Autodesk Inventor part; units mm, degrees
ref_plane "YZ Plane" through (0, 0, 0) normal (1, 0, 0) x (0, 1, 0)
ref_plane "XZ Plane" through (0, 0, 0) normal (0, 1, 0) x (-1, 0, 0)
ref_plane "XY Plane" through (0, 0, 0) normal (0, 0, 1) x (1, 0, 0)
sketch "Sketch1" plane through (0, 0, 0) normal (0, 0, 1) x (1, 0, 0)
  line L0 (0, 0) -> (-1016, 0)
  line L1 (-1016, 0) -> (-1016, 1016)
  line L2 (-1016, 1016) -> (0, 1016)
  line L3 (0, 1016) -> (0, 0)
  line L4 (19.05, 1035.05) -> (-1035.05, 1035.05)
  line L5 (-1035.05, 1035.05) -> (-1035.05, -19.05)
  line L6 (-1035.05, -19.05) -> (19.05, -19.05)
  line L7 (19.05, -19.05) -> (19.05, 1035.05)
  line L8 (-685.8, 1016) -> (-685.8, 1035.05)
  line L9 (-330.2, 1016) -> (-330.2, 1035.05)
  line L10 (-685.8, -19.05) -> (-685.8, 0)
  line L11 (-330.2, -19.05) -> (-330.2, 0)
  line L12 (0, 330.2) -> (19.05, 330.2)
  line L13 (0, 685.8) -> (19.05, 685.8)
  line L14 (-1016, 685.8) -> (-1035.05, 685.8)
  line L15 (-1016, 330.2) -> (-1035.05, 330.2)
  point P0 (-1644.65, 1016)
  point P1 (-1644.65, 1035.05)
  point P2 (-387.35, 1016)
  point P3 (-387.35, 1035.05)
  point P4 (-685.8, -19.05)
  point P5 (-685.8, 0)
  point P6 (-330.2, 0)
  point P7 (-330.2, -19.05)
  dimension "d0" = 1016
  dimension "d1" = 1016
  dimension "d2" = 19.05
  dimension "d5" = 355.6
  dimension "d7" = 355.6
  dimension "d10" = 349.25
  dimension "d11" = 349.25
  dimension "d12" = 355.6
  dimension "d13" = 349.25
  dimension "d14" = 349.25
  dimension "d15" = 349.25
  dimension "d18" = 349.25
extrude "Extrusion1" add sketch "Sketch1" along normal blind 19.05 contours L0 L1 L2 L3 | L11 L6 L10 L0 | L3 L13 L7 L12 | L15 L5 L14 L1 | L2 L8 L4 L9
properties part number "Final Product backplate"
Read the model definition and answer for the solid it produces. Units are mm, in the model's axes. Coordinates: 2 decimals unless noted, no trailing zeros. Loops run counter-clockwise (first coordinate to the right, second up) from the corner with the lowest first, then second, coordinate; pieces in that order, holes last.
Q1. Consider probe 1 along Y at (x, z) = (-134.5, 5.5); probe 2 along X at (y, z) = (924.5, 6.5). Determine where each line is inside the solid, lowest interval first.
Q2. The part is cut by section B-B on x = -757.5. Write down the section's boundary in (y, z).
Q3. The part is cut by section A-A on z = 12. Write down the section's boundary in (x, y).
Q4. Each of these flat-tipped pins is pushed along its axis until it touches: pin 1 Ø10 at (y, z) = (280, 4.5) entering from -X; pin 2 Ø9.5 at (x, z) = (10, 13.5) entering from -Y; pin 3 Ø1.5 at (x, z) = (-318.5, 5.5) entering from -Y. Where does it stop, or does it pass through?
Q5. The part is cut by section C-C on y = 74. Write down the section's boundary in (x, z), and give its area (3 significant figures).
Results below:
1. probe 1: y = 0 to 1016
1. probe 2: x = -1016 to 0
2. outline: (0, 0) - (1016, 0) - (1016, 19.05) - (0, 19.05) - close
3. outline: (-1035.05, 330.2) - (-1016, 330.2) - (-1016, 0) - (-685.8, 0) - (-685.8, -19.05) - (-330.2, -19.05) - (-330.2, 0) - (0, 0) - (0, 330.2) - (19.05, 330.2) - (19.05, 685.8) - (0, 685.8) - (0, 1016) - (-330.2, 1016) - (-330.2, 1035.05) - (-685.8, 1035.05) - (-685.8, 1016) - (-1016, 1016) - (-1016, 685.8) - (-1035.05, 685.8) - close
4. pin 1: stops at x = -1016
4. pin 2: stops at y = 330.2
4. pin 3: stops at y = 0
5. outline: (-1016, 0) - (0, 0) - (0, 19.05) - (-1016, 19.05) - close
5. area: 19,400 mm2
